Geometry: final body of the model. Coordinates: model frame, mm. A direction names the side the tool comes from. Coordinates: 2 decimals unless noted, no trailing zeros. Write each loop counter-clockwise with the first axis right and the second up, starting at its lowest first coordinate (ties: lowest second). Pieces come first, ordered by that corner, then holes. Notation, with made-up numbers: (33, -25.5) -> (75, -25.5) arc R25 ccw to (75, 10.5) -> close; hole circle Ø1 at (-5.75, 70). An arc over 180 degrees is marked (long way). One line per item, written item: value.
```python
from build123d import *

# Parameters (mm, degrees)
SKETCH_R        = 43
PAD_DEPTH       = 3
SKETCH001_R     = 43
SKETCH001_R_2   = 40
PAD001_DEPTH    = 11
SKETCH002_R     = 12.4
POCKET_DEPTH    = 5
SKETCH003_R     = 15
SKETCH003_R_2   = 12.4
PAD002_DEPTH    = 13
SKETCH004_R     = 15
SKETCH004_R_2   = 6
PAD003_DEPTH    = 3
SKETCH005_R     = 15
SKETCH005_R_2   = 7.75
PAD004_DEPTH    = 8
CHAMFER_SIZE    = 1.5
CHAMFER001_SIZE = 1.5
CHAMFER002_SIZE = 1.5
CHAMFER003_SIZE = 1.5


with BuildPart() as part:
    # Sketch → Pad (new body)
    with BuildSketch(Plane.XY):
        Circle(SKETCH_R)
    extrude(amount=PAD_DEPTH)

    # Sketch001 (on Face3 of Pad) → Pad001 (join)
    with BuildSketch(Plane.XY.offset(3)):
        Circle(SKETCH001_R)
        Circle(SKETCH001_R_2, mode=Mode.SUBTRACT)
    extrude(amount=PAD001_DEPTH)

    # Sketch002 (on Face6 of Pad001) → Pocket (cut)
    with BuildSketch(Plane.XY.offset(3)):
        Circle(SKETCH002_R)
    extrude(amount=-POCKET_DEPTH, mode=Mode.SUBTRACT)

    # Sketch003 (on Face2 of Pocket) → Pad002 (join)
    with BuildSketch(Plane(origin=(0, 0, 0), x_dir=(1, 0, 0), z_dir=(0, 0, -1))):
        Circle(SKETCH003_R)
        Circle(SKETCH003_R_2, mode=Mode.SUBTRACT)
    extrude(amount=PAD002_DEPTH)

    # Sketch004 (on Face6 of Pad002) → Pad003 (join)
    with BuildSketch(Plane(origin=(0, 0, -13), x_dir=(1, 0, 0), z_dir=(0, 0, -1))):
        Circle(SKETCH004_R)
        Circle(SKETCH004_R_2, mode=Mode.SUBTRACT)
    extrude(amount=PAD003_DEPTH)

    # Sketch005 (on Face8 of Pad003) → Pad004 (join)
    with BuildSketch(Plane(origin=(0, 0, -16), x_dir=(1, 0, 0), z_dir=(0, 0, -1))):
        Circle(SKETCH005_R)
        with Locations((0, -0.177664)):
            Circle(SKETCH005_R_2, mode=Mode.SUBTRACT)
    extrude(amount=PAD004_DEPTH)

    # Chamfer
    chamfer_edges = [part.edges().sort_by_distance(p)[0] for p in [
        (-15, 0, -24),
    ]]
    chamfer(chamfer_edges, length=CHAMFER_SIZE)

    # Chamfer001
    chamfer001_edges = [part.edges().sort_by_distance(p)[0] for p in [
        (-7.75, 0.177664, -24),
    ]]
    chamfer(chamfer001_edges, length=CHAMFER001_SIZE)

    # Chamfer002
    chamfer002_edges = [part.edges().sort_by_distance(p)[0] for p in [
        (-12.4, 0, 3),
    ]]
    chamfer(chamfer002_edges, length=CHAMFER002_SIZE)

    # Chamfer003
    chamfer003_edges = [part.edges().sort_by_distance(p)[0] for p in [
        (-40, 0, 14),
    ]]
    chamfer(chamfer003_edges, length=CHAMFER003_SIZE)


solid = part.part
```
(1) Section B-B (z = -11). Return the cut outline in (x, y), then the cut area to 3 significant figures.
Responses:
outline: circle Ø30 at (0, 0); hole circle Ø24.8 at (0, 0)
area: 224 mm2
(2) First-contact query: pin 1 (2 mm diameter, centred on x = 33.5, z = 3, fed in from +Y); pin 2 (12 mm diameter, centred on y = -29.5, z = -9, fed in from +X); pin 3 (3 mm diameter, centred on x = -2.5, z = 9, fed in from -Y); pin 4 (4 mm diameter, centred on x = -11, y = 12, fed in from +Z). Flat tips, straight axial feed; report the tip coordinate or a pass-through.
Responses:
pin 1: stops at y = 28.16
pin 2: passes through
pin 3: stops at y = -42.99
pin 4: stops at z = 3
(3) Pull-direction query (Y, two-part tool) for faces 4 (the flat face through (9, -3, -24)), 5 (the cylindrical face through (-5.598, 42.634, 6.902)), 6 (the cylindrical face through (-1.68, 7.743, -19.204)); classes: released by +Y, released by -Y, zero draft, split by the parting line, or undercut.
Responses:
face 4: zero draft
face 5: split by the parting line
face 6: undercut
(4) Reachability of faces 1 (the flat face through (2, 6, -16)), 2 (the cylindrical face through (-6, 0, -14)), 3 (the flat face through (-1, -17, 3)) from +Z, -Z, +X, -X, +Y, -Y: full face, straight path, thin tool, end or side. Return the list, or none.
Responses:
face 1: -Z
face 2: +Z, -Z
face 3: +Z
(5) Line query: line 1 (Y direction, x = 0, z = -17.25); line 2 (Y direction, x = 0, z = -14); line 3 (Z direction, x = 16, y = 26). Output: solid intervals per line, ascending. Write a range as [from, to].
Responses:
line 1: y = [-15, -7.57], [7.93, 15]
line 2: y = [-15, -6], [6, 15]
line 3: z = [0, 3]
